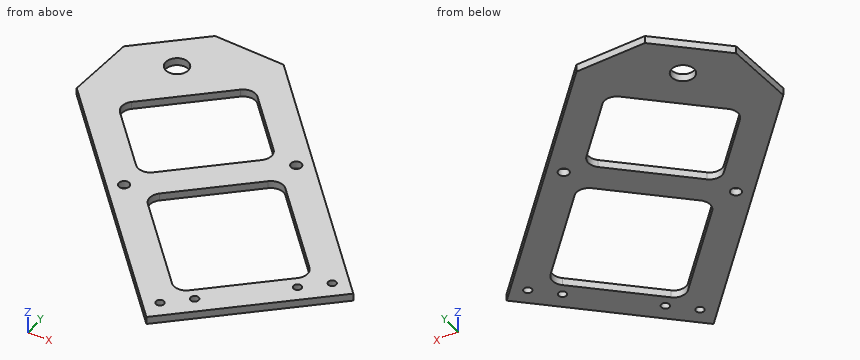
from build123d import *

# Parameters (mm, degrees)
SKETCH_1_R      = 2.1
SKETCH_1_R_2    = 4.5
SKETCH_1_R_3    = 1.6
EXTRUDE_1_DEPTH = 3


with BuildPart() as part:
    # 草图1 → 凸台-拉伸1 (new body)
    with BuildSketch(Plane.XY):
        Polygon((-324.62596071, -164.077614251), (-272.3024403, -115.202168351), (-361.042775034, -20.201363137), (-389.310642718, -19.238213832), (-412.403146139, -40.808941352), (-413.366295444, -69.076809037), align=None)
        with Locations((-327.200821851, -65.220494679)):
            Circle(SKETCH_1_R, mode=Mode.SUBTRACT)
        with Locations((-370.755037164, -105.904525064)):
            Circle(SKETCH_1_R, mode=Mode.SUBTRACT)
        with Locations((-391.163719404, -40.400588623)):
            Circle(SKETCH_1_R_2, mode=Mode.SUBTRACT)
        with Locations((-325.019633878, -154.866478521)):
            Circle(SKETCH_1_R_3, mode=Mode.SUBTRACT)
        with Locations((-316.250328782, -146.675063007)):
            Circle(SKETCH_1_R_3, mode=Mode.SUBTRACT)
        with Locations((-290.234723661, -122.373863649)):
            Circle(SKETCH_1_R_3, mode=Mode.SUBTRACT)
        with Locations((-281.465418565, -114.182448135)):
            Circle(SKETCH_1_R_3, mode=Mode.SUBTRACT)
        with BuildLine():
            Line((-320.394194004, -143.703803843), (-292.917038034, -118.037368566))
            ThreePointArc((-292.917038034, -118.037368566), (-291.333027599, -114.553753794), (-292.676250708, -110.970401645))
            Line((-292.676250708, -110.970401645), (-323.394058885, -78.085507532))
            ThreePointArc((-323.394058885, -78.085507532), (-326.877673657, -76.501497097), (-330.461025806, -77.844720206))
            Line((-330.461025806, -77.844720206), (-357.938181776, -103.511155483))
            ThreePointArc((-357.938181776, -103.511155483), (-359.522192211, -106.994770255), (-358.178969102, -110.578122404))
            Line((-358.178969102, -110.578122404), (-327.461160925, -143.463016517))
            ThreePointArc((-327.461160925, -143.463016517), (-323.977546152, -145.047026952), (-320.394194004, -143.703803843))
        make_face(mode=Mode.SUBTRACT)
        with BuildLine():
            Line((-366.12959729, -94.741850386), (-338.65244132, -69.075415109))
            ThreePointArc((-338.65244132, -69.075415109), (-337.068430885, -65.591800337), (-338.411653994, -62.008448188))
            Line((-338.411653994, -62.008448188), (-358.890192778, -40.085185447))
            ThreePointArc((-358.890192778, -40.085185447), (-362.373807551, -38.501175012), (-365.957159699, -39.84439812))
            Line((-365.957159699, -39.84439812), (-393.434315669, -65.510833397))
            ThreePointArc((-393.434315669, -65.510833397), (-395.018326104, -68.99444817), (-393.675102995, -72.577800318))
            Line((-393.675102995, -72.577800318), (-373.196564211, -94.50106306))
            ThreePointArc((-373.196564211, -94.50106306), (-369.712949438, -96.085073495), (-366.12959729, -94.741850386))
        make_face(mode=Mode.SUBTRACT)
    extrude(amount=EXTRUDE_1_DEPTH)


solid = part.part
The model under review builds one solid part; all positions refer to its coordinate system, in mm. Give positions to 0.01 mm unless a question says otherwise; leave off trailing zeros. Order: outer loops, then holes, each group sorted by start corner. A loop starts at its lowest first (then second) coordinate and runs counter-clockwise, first axis right, second up. Notation, with made-up numbers: (29, -29.5) -> (87, -29.5) arc R32 cw to (87, -2.5) -> close; hole circle Ø3 at (32, 14). An arc over 180 degrees is marked (long way). Write item = value, one per line. Start each with the question number.
(1) Take a section at B-B (z = 2.3). State how many separate pieces and enclosed holes the cut face has, plus the area to 3 significant figures.
(2) For pin 1 Ø2.5 at (x, y) = (-281.47, -114.18) entering from -Z; pin 2 Ø1.5 at (y, z) = (-126.5, 2) entering from +X, all flat-tipped, find the tip position at first contact; note any pin that passes through.
(3) Take a section at C-C (y = -135). Write out the cut boundary in (x, z), plus the area to 3 significant figures.
(4) Take a section at A-A (x = -380.5). Write out the cut boundary in (y, z).
(5) For L1, parallel to X at y = -66, z = 0.45; L2, parallel to X at y = -79, z = 0.4; L3, parallel to Y at x = -353.5, z = 2, list the stretches that pass through material, from the lowest coordinate up. Write a range as from..to.
(6) Take a section at D-D (x = -352). Write out the cut boundary in (y, z), plus the area to 3 significant figures.
Returned:
q1.separate_pieces = 1
q1.enclosed_holes = 9
q1.area = 5,740 mm²
q2.pin_1 = through
q2.pin_2 = -283.59
q3.outline = (-351.79, 0) -> (-335.37, 0) -> (-335.37, 3) -> (-351.79, 3) -> close; (-311.08, 0) -> (-293.5, 0) -> (-293.5, 3) -> (-311.08, 3) -> close
q3.area = 102 mm²
q4.outline = (-104.26, 0) -> (-86.68, 0) -> (-86.68, 3) -> (-104.26, 3) -> close; (-53.43, 0) -> (-19.54, 0) -> (-19.54, 3) -> (-53.43, 3) -> close
q5.L1 = -413.26..-393.89, -337.1..-329.15, -325.25..-318.26
q5.L2 = -404.1..-387.68, -349.28..-331.7, -322.54..-306.12
q5.L3 = -133.17..-115.59, -99.37..-82.94, -45.86..-28.28
q6.outline = (-134.77, 0) -> (-117.19, 0) -> (-117.19, 3) -> (-134.77, 3) -> close; (-97.96, 0) -> (-81.54, 0) -> (-81.54, 3) -> (-97.96, 3) -> close; (-47.46, 0) -> (-29.88, 0) -> (-29.88, 3) -> (-47.46, 3) -> close
q6.area = 155 mm²
